Autodesk Inventor part; units mm, degrees
ref_plane "YZ Plane" through (0, 0, 0) normal (1, 0, 0) x (0, 1, 0)
ref_plane "XZ Plane" through (0, 0, 0) normal (0, 1, 0) x (-1, 0, 0)
ref_plane "XY Plane" through (0, 0, 0) normal (0, 0, 1) x (1, 0, 0)
sketch "Sketch1" plane through (0, 0, 0) normal (0, 0, 1) x (1, 0, 0)
  line L0 (2.4765, 2.4985) -> (2.4765, -2.4985)
  line L1 (-2.4765, 2.4985) -> (-2.4765, -2.4985)
  arc A0 (-2.4765, -2.4985) -> (2.4765, -2.4985) centre (0, 0) ccw
  arc A1 (2.4765, 2.4985) -> (-2.4765, 2.4985) centre (0, 0) ccw
  line L2 (4.572, 4.2217) -> (4.572, -4.2217)
  line L3 (-4.572, 4.2217) -> (-4.572, -4.2217)
  arc A2 (-4.572, -4.2217) -> (4.572, -4.2217) centre (0, 0) ccw
  arc A3 (4.572, 4.2217) -> (-4.572, 4.2217) centre (0, 0) ccw
  dimension "d2" = 2.4765
  dimension "d3" = 4.953
  dimension "d6" = 4.572
  dimension "d7" = 9.144
  dimension "d8" = 3.5179
  dimension "d9" = 3.5179
  dimension "d10" = 6.223
  dimension "d11" = 6.223
extrude "Extrusion1" add sketch "Sketch1" along normal blind 45.72
properties part number "Motor Shaft Extension"
Source: CAD feature listing. Evaluate the final solid. Frame: model axes, mm. A direction names the side the tool comes from. Round coordinates to 2 decimals unless told otherwise and drop trailing zeros. Write each loop counter-clockwise with the first axis right and the second up, starting at its lowest first coordinate (ties: lowest second). Pieces come first, ordered by that corner, then holes. Notation, with made-up numbers: M 62.5,87 L 91.5,87 A8 cw 91.5,97 Z; hole C -34.5,31.5 d2. An arc over 180 degrees is marked long. One line per item, written item: value. Start each with the question number.
Item 1: Section query A-A (x = 0). Return the cut outline in (y, z).
Item 2: Section query B-B (y = -0.25). Return the cut outline in (x, z).
Item 3: Set-up query: faces 1 (the flat face through (-4.572, 0, 23)), 2 (the flat face through (2.476, 0, 23)). Return all of +Z, -Z, +X, -X, +Y, -Y with unobstructed straight access to the full face (end or side cutting, diameter ignored); none if empty.
Item 4: Mould query, pull axis Y, two halves, no side actions, for faces 3 (the flat face through (3, 0, 0)), 4 (the cylindrical face through (0.072, -6.223, 22.54)), 5 (the cylindrical face through (0.038, -3.518, 22.54)). Classes: pulls with the +Y half, pulls with the -Y half, needs draft (parallel to the pull), parting line crosses it, or undercut.
Item 5: Pin query (flat end, axial travel): pin 1 (3 mm diameter, centred on x = -1.5, y = 2, fed in from +Z); pin 2 (1 mm diameter, centred on x = -2, z = 33.5, fed in from +Y). Return the tip coordinate at first contact, or that it passes through.
Item 6: Ray query, L1, parallel to X at y = -0.25, z = 2.5; L2, parallel to Y at x = -2.25, z = 30.5; L3, parallel to Y at x = 1.5, z = 4.5. Return the intervals inside material, ascending. Write a range as from..to.
Item 7: Section query D-D (y = 5). Return the cut outline in (x, z).
Item 8: Section query C-C (z = 28.5). Return the cut outline in (x, y).
Result set:
1. outline: M -6.22,0 L -3.52,0 L -3.52,45.72 L -6.22,45.72 Z; M 3.52,0 L 6.22,0 L 6.22,45.72 L 3.52,45.72 Z
2. outline: M -4.57,0 L -2.48,0 L -2.48,45.72 L -4.57,45.72 Z; M 2.48,0 L 4.57,0 L 4.57,45.72 L 2.48,45.72 Z
3. face 1: +Z, -Z, -X, +Y, -Y
3. face 2: +Z, -Z
4. face 3: needs draft
4. face 4: pulls with the -Y half
4. face 5: undercut
5. pin 1: stops at z = 45.72
5. pin 2: stops at y = 6.04
6. L1: x = -4.57..-2.48, 2.48..4.57
6. L2: y = -5.8..-2.7, 2.7..5.8
6. L3: y = -6.04..-3.18, 3.18..6.04
7. outline: M -3.7,0 L 3.7,0 L 3.7,45.72 L -3.7,45.72 Z
8. outline: M -4.57,-4.22 A6.22 ccw 4.57,-4.22 L 4.57,4.22 A6.22 ccw -4.57,4.22 Z; hole M -2.48,-2.5 A3.52 ccw 2.48,-2.5 L 2.48,2.5 A3.52 ccw -2.48,2.5 Z
